from build123d import *

# Parameters (mm, degrees)
BOSS_EXTRUDE1_DEPTH = 13.6
DEBURS_SIZE         = 0.5


with BuildPart() as part:
    # Sketch1 → Boss-Extrude1 (new body)
    with BuildSketch(Plane.XY):
        with BuildLine():
            Line((-65.5, 45.5), (-65.5, -45.5))
            ThreePointArc((-65.5, -45.5), (-64.474873734, -47.974873734), (-62, -49))
            Line((-62, -49), (62, -49))
            ThreePointArc((62, -49), (64.474873734, -47.974873734), (65.5, -45.5))
            Line((65.5, -45.5), (65.5, 45.5))
            ThreePointArc((65.5, 45.5), (64.474873734, 47.974873734), (62, 49))
            Line((62, 49), (-62, 49))
            ThreePointArc((-62, 49), (-64.474873734, 47.974873734), (-65.5, 45.5))
        make_face()
        with BuildLine():
            Line((-56.9, 44.6), (56.9, 44.6))
            ThreePointArc((56.9, 44.6), (58.314213562, 44.014213562), (58.9, 42.6))
            Line((58.9, 42.6), (58.9, -42.6))
            ThreePointArc((58.9, -42.6), (58.314213562, -44.014213562), (56.9, -44.6))
            Line((56.9, -44.6), (-56.9, -44.6))
            ThreePointArc((-56.9, -44.6), (-58.314213562, -44.014213562), (-58.9, -42.6))
            Line((-58.9, -42.6), (-58.9, 42.6))
            ThreePointArc((-58.9, 42.6), (-58.314213562, 44.014213562), (-56.9, 44.6))
        make_face(mode=Mode.SUBTRACT)
    extrude(amount=BOSS_EXTRUDE1_DEPTH)

    # Deburs
    deburs_edges = [part.edges().sort_by_distance(p)[0] for p in [
        (58.314213562, 44.014213562, 0),
        (0, 44.6, 0),
        (-58.314213562, 44.014213562, 0),
        (-58.9, 0, 0),
        (-58.314213562, -44.014213562, 0),
        (0, -44.6, 0),
        (-64.474873734, 47.974873734, 13.6),
        (-64.474873734, 47.974873734, 0),
        (-65.5, 0, 13.6),
        (-65.5, 0, 0),
        (-64.474873734, -47.974873734, 13.6),
        (-64.474873734, -47.974873734, 0),
        (0, -49, 13.6),
        (0, -49, 0),
        (64.474873734, -47.974873734, 13.6),
        (64.474873734, -47.974873734, 0),
        (65.5, 0, 13.6),
        (65.5, 0, 0),
        (58.314213562, -44.014213562, 0),
        (64.474873734, 47.974873734, 13.6),
        (64.474873734, 47.974873734, 0),
        (0, 49, 13.6),
        (0, 49, 0),
        (58.314213562, -44.014213562, 13.6),
        (0, -44.6, 13.6),
        (-58.314213562, -44.014213562, 13.6),
        (-58.9, 0, 13.6),
        (-58.314213562, 44.014213562, 13.6),
        (0, 44.6, 13.6),
        (58.314213562, 44.014213562, 13.6),
        (58.9, 0, 13.6),
        (58.9, 0, 0),
    ]]
    chamfer(deburs_edges, length=DEBURS_SIZE)


solid = part.part
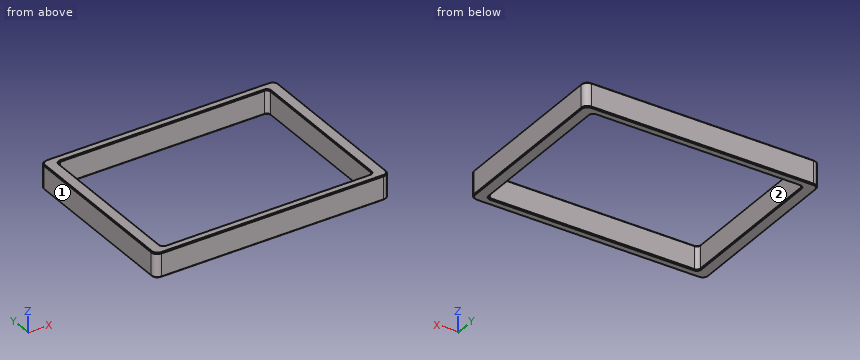
Model file for the job. Use its own axes, mm. Face numbers are marked on the shaded views. A direction names the side the tool comes from. Round coordinates to 2 decimals unless told otherwise and drop trailing zeros. Order: outer loops, then holes, each group sorted by start corner. A loop starts at its lowest first (then second) coordinate and runs counter-clockwise, first axis right, second up.
(1) Band-saw the part on C-C (x = 21.5). List the corners of the cut face in (y, z).
(2) 3-axis set-ups, long thin cutter, end or side, ignore diameter. For the marked faces 1 and 2: which of +Z, -Z, +X, -X, +Y, -Y reach the whole face in a straight line?
(3) Band-saw the part on A-A (y = -36.5). List the corners of the cut face in (x, z), then the cut area to 3 significant figures.
(4) Drill centre lines: line 1 (X direction, y = 3, z = 11.75); line 2 (Y direction, x = -33.5, z = 6.5); line 3 (Y direction, x = -58, z = 1.25). Where is each one in solid material? Low to high.
(5) Band-saw the part on B-B (z = 11.75). List the corners of the cut face in (x, y).
Verdict:
1. outline: (-49, 0.5) - (-48.5, 0) - (-45.1, 0) - (-44.6, 0.5) - (-44.6, 13.1) - (-45.1, 13.6) - (-48.5, 13.6) - (-49, 13.1) - close; (44.6, 0.5) - (45.1, 0) - (48.5, 0) - (49, 0.5) - (49, 13.1) - (48.5, 13.6) - (45.1, 13.6) - (44.6, 13.1) - close
2. face 1: +Z, -Z, -X, +Y, -Y
2. face 2: +Z, -Z
3. outline: (-65.5, 0.5) - (-65, 0) - (-59.4, 0) - (-58.9, 0.5) - (-58.9, 13.1) - (-59.4, 13.6) - (-65, 13.6) - (-65.5, 13.1) - close; (58.9, 0.5) - (59.4, 0) - (65, 0) - (65.5, 0.5) - (65.5, 13.1) - (65, 13.6) - (59.4, 13.6) - (58.9, 13.1) - close
3. area: 179 mm2
4. line 1: x = -65.5 to -58.9, 58.9 to 65.5
4. line 2: y = -49 to -44.6, 44.6 to 49
4. line 3: y = -49 to -44.27, 44.27 to 49
5. outline: (-65.5, -45.5) arc R3.5 ccw to (-62, -49) - (62, -49) arc R3.5 ccw to (65.5, -45.5) - (65.5, 45.5) arc R3.5 ccw to (62, 49) - (-62, 49) arc R3.5 ccw to (-65.5, 45.5) - close; hole (-58.9, -42.6) arc R2 ccw to (-56.9, -44.6) - (56.9, -44.6) arc R2 ccw to (58.9, -42.6) - (58.9, 42.6) arc R2 ccw to (56.9, 44.6) - (-56.9, 44.6) arc R2 ccw to (-58.9, 42.6) - close
